Could you check a few things on this model? Use its own coordinates, in mm. A direction names the side the tool comes from. Coordinates: 2 decimals unless noted, no trailing zeros. Loops run counter-clockwise (first coordinate to the right, second up) from the corner with the lowest first, then second, coordinate; pieces in that order, holes last. Notation, with made-up numbers: (-22, 58) -> (31, 58) arc R23 ccw to (31, 84) -> close; hole circle Ø9 at (63.25, 64.5). An arc over 180 degrees is marked (long way). One line per question, with ' | ' between items.
```python
from build123d import *

# Parameters (mm, degrees)
BOSS_EXTRUDE1_DEPTH = 1.5875
SKETCH2_W           = 36.068
SKETCH2_H           = 1.5875
BOSS_EXTRUDE2_DEPTH = 21.2725
SKETCH3_W           = 1.5875
SKETCH3_H           = 25.654
BOSS_EXTRUDE3_DEPTH = 6.35
FILLET1_R           = 3.175
HOLE1_D             = 5.08
HOLE1_DEPTH         = 15.875
HOLE2_D             = 2.8448
SKETCH9_W           = 48.514
SKETCH9_H           = 25.908
BOSS_EXTRUDE4_DEPTH = 30.988
HOLE3_D             = 2.8448
LPATTERN1_COUNT     = 2
LPATTERN1_PITCH     = 10.16
SKETCH12_W          = 1.4224
SKETCH12_H          = 36.3855
LPATTERN2_COUNT     = 2
LPATTERN2_PITCH     = 28.575


with BuildPart() as part:
    # Sketch1 → Boss-Extrude1 (new body)
    with BuildSketch(Plane(origin=(0, 0, 0), x_dir=(1, 0, 0), z_dir=(0, 1, 0))):
        Polygon((0, 0), (0, -25.4), (13.2588, -56.388), (31.9532, -56.388), (31.9532, -49.3268), (80.4672, -49.3268), (80.4672, 0), align=None)
    extrude(amount=BOSS_EXTRUDE1_DEPTH)

    # Sketch2 → Boss-Extrude2 (add)
    with BuildSketch(Plane.XZ):
        with Locations((18.034, 0.79375)):
            Rectangle(SKETCH2_W, SKETCH2_H)
    extrude(amount=BOSS_EXTRUDE2_DEPTH)

    # Sketch3 → Boss-Extrude3 (add)
    with BuildSketch(Plane.XY.offset(1.5875)):
        with Locations((35.27425, -21.971)):
            Rectangle(SKETCH3_W, SKETCH3_H)
        with Locations((0.79375, -21.971)):
            Rectangle(SKETCH3_W, SKETCH3_H)
    extrude(amount=BOSS_EXTRUDE3_DEPTH)

    # Fillet1
    # the kernel refuses this fillet: 3.175 mm, written as the material it adds along each edge
    with BuildSketch(Plane(origin=(34.4805, -21.2725, 1.5875), x_dir=(0, 0, -1), z_dir=(1, 0, 0)), Plane(origin=(0, -21.2725, 1.5875), x_dir=(0, 0, -1), z_dir=(1, 0, 0))) as fillet1_piece_1:
        with BuildLine():
            CenterArc((3.175, -2.749630657), FILLET1_R, 120, 60)
            Line((0, -2.749630657), (0, 0))
            Line((0, 0), (1.5875, 0))
        make_face()
    extrude(amount=1.5875)
    # the kernel refuses this fillet: 3.175 mm, written as the material it takes off along each edge
    with BuildSketch(Plane(origin=(26.543, -34.798, 1.5875), x_dir=(0, 1, 0), z_dir=(1, 0, 0)), Plane(origin=(44.0055, -9.144, 7.9375), x_dir=(0, 0, -1), z_dir=(-1, 0, 0)), Plane(origin=(9.525, -34.798, 1.5875), x_dir=(0, 0, 1), z_dir=(-1, 0, 0)), Plane(origin=(9.525, -34.798, 7.9375), x_dir=(0, 1, 0), z_dir=(-1, 0, 0))) as fillet1_2_piece_1:
        with BuildLine():
            CenterArc((FILLET1_R, FILLET1_R), FILLET1_R, 180, 90)
            Line((0, FILLET1_R), (0, 0))
            Line((0, 0), (FILLET1_R, 0))
        make_face()
    extrude(amount=17.4625, mode=Mode.SUBTRACT)
    with BuildSketch(Plane(origin=(26.543, -34.798, 7.9375), x_dir=(0, 1, 0), z_dir=(1, 0, 0)), Plane(origin=(-7.9375, -9.144, 7.9375), x_dir=(0, 0, -1), z_dir=(1, 0, 0))) as fillet1_2_piece_2:
        with BuildLine():
            CenterArc((FILLET1_R, -FILLET1_R), FILLET1_R, 90, 90)
            Line((0, -FILLET1_R), (0, 0))
            Line((0, 0), (FILLET1_R, 0))
        make_face()
    extrude(amount=17.4625, mode=Mode.SUBTRACT)

    # Hole1
    with Locations(Plane(origin=(0, 0, 0), x_dir=(-1, 0, 0), z_dir=(0, 0, -1))):
        with Locations((-18.034, -9.8425)):
            Hole(HOLE1_D / 2, depth=HOLE1_DEPTH)

    # Hole2 (through all)
    with Locations(Plane(origin=(36.068, 3.937526914, -1.455484635), x_dir=(0, 0, -1), z_dir=(1, 0, 0))):
        with Locations((-6.217984635, -32.050026914)):
            Hole(HOLE2_D / 2)

    # Sketch9 → Boss-Extrude4 (add)
    with BuildSketch(Plane(origin=(0, 1.5875, 0), x_dir=(1, 0, 0), z_dir=(0, 1, 0))):
        with Locations((46.863, -25.7048)):
            Rectangle(SKETCH9_W, SKETCH9_H)
    extrude(amount=BOSS_EXTRUDE4_DEPTH)

    # Hole3 (through all)
    with Locations(Plane(origin=(0, 1.5875, 0), x_dir=(-1, 0, 0), z_dir=(0, 1, 0))):
        with Locations((-25.7175, 50.038)):
            hole3 = Hole(HOLE3_D / 2)

    # LPattern1: Hole3 ×2
    with Locations(*[(-i * LPATTERN1_PITCH, 0, 0) for i in range(1, LPATTERN1_COUNT)]):
        add(hole3, mode=Mode.SUBTRACT)

    # Sketch12 → Hole4 (revolve, cut)
    with BuildSketch(Plane(origin=(6.35, 1.5875, 25.4), x_dir=(0, 0, 1), z_dir=(1, 0, 0))):
        with Locations((0.7112, 18.19275)):
            Rectangle(SKETCH12_W, SKETCH12_H)
    hole4 = revolve(axis=Axis((6.35, -108.4125, 25.4), (0, 1, 0)), mode=Mode.SUBTRACT)

    # LPattern2: Hole4 ×2
    with Locations(*[(i * LPATTERN2_PITCH, 0, 0) for i in range(1, LPATTERN2_COUNT)]):
        add(hole4, mode=Mode.SUBTRACT)


solid = part.part
```
Q1. For pin 1 (5 mm diameter, centred on x = 61, y = 22, fed in from -Z); pin 2 (10 mm diameter, centred on y = -5.5, z = 11.5, fed in from -X); pin 3 (6.5 mm diameter, centred on x = 18.03, y = -9.84, fed in from +Z); pin 4 (4.5 mm diameter, centred on x = 15.56, z = 50.04, fed in from -Y), each with a flat end and sliding along its axis, tell me the tip position at first contact or that it passes through.
Values follow:
pin 1: stops at z = 12.75 | pin 2: passes through | pin 3: stops at z = 1.59 | pin 4: stops at y = 0
Q2. Imagine slicing it at C-C on z = 35.5. Write out the boundary of the cut face in (x, y).
Values follow:
outline: (4.32, 0) -> (80.47, 0) -> (80.47, 1.59) -> (71.12, 1.59) -> (71.12, 32.58) -> (22.61, 32.58) -> (22.61, 1.59) -> (4.32, 1.59) -> close
Q3. Imagine slicing it at A-A on x = 45. Write out the boundary of the cut face in (y, z).
Values follow:
outline: (0, 0) -> (1.59, 0) -> (1.59, 12.75) -> (32.58, 12.75) -> (32.58, 38.66) -> (1.59, 38.66) -> (1.59, 49.33) -> (0, 49.33) -> close
Q4. For faces 5 (the face through (35, 1.588, 25)), 6 (the face through (34.48, -22, 5)), 7 (the face through (0.783, -10.049, 6.983)), 8 (the face through (36.068, -17, 4)), 9 (the face through (22.606, 17, 26)), which set-ups out of +Z, -Z, +X, -X, +Y, -Y let a thin tool reach every point of the face, with its end or its side?
Values follow:
face 5: -Y | face 6: +Z, -Y | face 7: +Z, +X, -X | face 8: +Z, -Z, +X, -Y | face 9: +Z, -Z, -X, +Y
Q5. Imagine slicing it at B-B on x = 25.5. Write out the boundary of the cut face in (y, z).
Values follow:
outline: (-21.27, 0) -> (1.59, 0) -> (1.59, 12.75) -> (32.58, 12.75) -> (32.58, 38.66) -> (1.59, 38.66) -> (1.59, 48.63) -> (0, 48.63) -> (0, 1.59) -> (-21.27, 1.59) -> close; (0, 51.44) -> (1.59, 51.44) -> (1.59, 56.39) -> (0, 56.39) -> close
Q6. We'd pull the mould along Z, two halves only. Please class faces 1 (the face through (35.285, -10.099, 7.032)), 2 (the face through (5.805, 0.783, 26.714)), 3 (the face through (14.51, 0.78, 51)), 4 (the face through (40, 0, 28)): released by +Z, released by -Z, zero draft, split by the parting line, or undercut.
Values follow:
face 1: released by +Z | face 2: undercut | face 3: undercut | face 4: zero draft
Q7. Imagine slicing it at D-D on y = 6. Write out the boundary of the cut face in (x, z).
Values follow:
outline: (22.61, 12.75) -> (71.12, 12.75) -> (71.12, 38.66) -> (22.61, 38.66) -> close
Q8. Please list where these lines run through material, in increasing order: L1, parallel to Y at x = 76, z = 31.5; L2, parallel to Y at x = 64.5, z = 31; L3, parallel to Z at x = 35.5, y = 14.5. Write a range as [from, to].
Values follow:
L1: y = [0, 1.59] | L2: y = [0, 32.58] | L3: z = [12.75, 38.66]
